Part print with two shaded views. Sizes in mm from the minimum x, y, z corner. A direction names the side the tool comes from. Coordinates: 2 decimals unless noted, no trailing zeros. Loops run counter-clockwise (first coordinate to the right, second up) from the corner with the lowest first, then second, coordinate; pieces in that order, holes last. Notation, with made-up numbers: (63.5, 42.25) -> (68.5, 42.25) arc R19 cw to (68.5, 69.25) -> close; hole circle Ø4 at (78, -15.5). An arc over 180 degrees is marked (long way). Return JSON: item names as keys, results as strings. Group by question number.
(1) Flat gauge pins, fed straight in: pin 1 Ø6 at (x, z) = (9, 4.5) entering from +Y; pin 2 Ø5 at (x, y) = (6.5, 7.5) entering from +Z; pin 3 Ø1 at (x, y) = (6.5, 4.5) entering from +Z. Where does each tip first touch, or does it go through?
(2) Tool access for the marked faces 1 and 2: list every direction of +Z, -Z, +X, -X, +Y, -Y with a clear straight run to the whole face (end or side of a thin tool).
(3) Saw through at B-B on y = 17. Write the cut outline in (x, z).
(4) Probe L1, parallel to Y at x = 5.08, z = 3.5 (1 decimal); L2, parallel to Z at x = 8.25, y = 16; L3, parallel to Z at x = 2.5, y = 6.5. List the from-to ranges inside material, lowest first.
(5) Mould opens along Y. For the marked faces 3, 4 and 5 say: pulls with the +Y half, pulls with the -Y half, needs draft (parallel to the pull), parting line crosses it, or undercut.
(6) Saw through at C-C on y = 10. Write the cut outline in (x, z), then the cut area to 3 significant figures.
(7) Saw through at A-A on z = 6. Write the cut outline in (x, y).
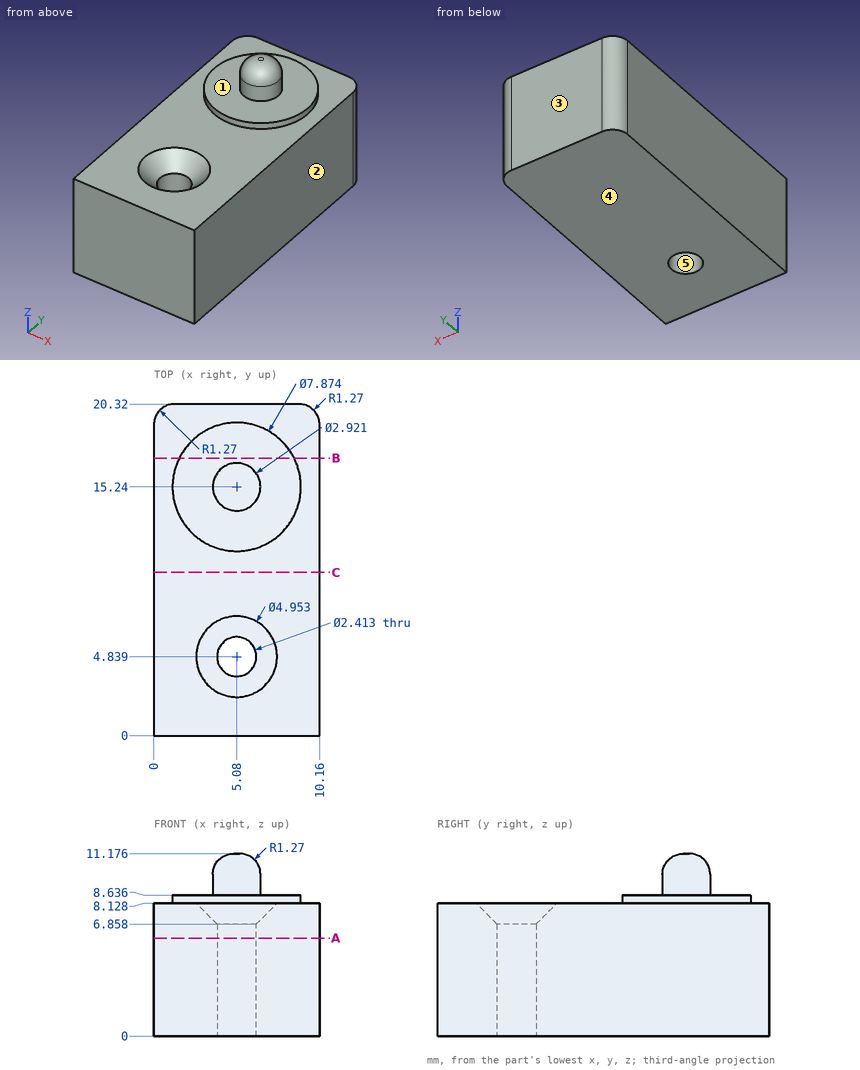
Geometry results:
{
 "1": {"pin 1": "y = 20.32", "pin 2": "z = 8.13", "pin 3": "z = 7.61"},
 "2": {"face 1": "+Z", "face 2": "+Z, -Z, +X, +Y, -Y"},
 "3": {"outline": "(0, 0) -> (10.16, 0) -> (10.16, 8.13) -> (8.6, 8.13) -> (8.6, 8.64) -> (1.56, 8.64) -> (1.56, 8.13) -> (0, 8.13) -> close"},
 "4": {"L1": "0 to 3.6, 6 to 20.3", "L2": "0 to 8.64", "L3": "0 to 8.13"},
 "5": {"face 3": "pulls with the +Y half", "face 4": "needs draft", "face 5": "undercut"},
 "6": {"outline": "(0, 0) -> (10.16, 0) -> (10.16, 8.13) -> (0, 8.13) -> close", "area": "82.6 mm²"},
 "7": {"outline": "(0, 0) -> (10.16, 0) -> (10.16, 19.05) arc R1.27 ccw to (8.89, 20.32) -> (1.27, 20.32) arc R1.27 ccw to (0, 19.05) -> close; hole circle Ø2.41 at (5.08, 4.84)"}
}
